Geometry check sheet. Reference: drawing and pictorial views, mm from the part's lowest x, y, z. A direction names the side the tool comes from. Coordinates: 2 decimals unless noted, no trailing zeros. Loops run counter-clockwise (first coordinate to the right, second up) from the corner with the lowest first, then second, coordinate; pieces in that order, holes last. Notation, with made-up numbers: (57, -30) -> (64, -30) arc R16 ccw to (64, 1) -> close; hole circle Ø3 at (-27.75, 43.25). An arc over 180 degrees is marked (long way). Answer as a JSON object with one key per item and string values. Group by question number.
Q1. Set-up check for the marked faces 1, 2 and 3: record each of +Z, -Z, +X, -X, +Y, -Y from which the full face is reachable in a straight line by a thin tool's end or side.
Q2. Cross-section at C-C on z = 3.2. Record the boundary of the cut face in (x, y), and give its area (3 significant figures).
Q3. Gauge pin test, flat ends, axial feed: pin 1 Ø1 at (x, z) = (6, 1.5) entering from +Y; pin 2 Ø1 at (x, z) = (2, 1) entering from +Y; pin 3 Ø2 at (y, z) = (15, 2) entering from +X. Record the tip position at first contact, or that the pin passes through.
Q4. Cross-section at D-D on z = 0.4. Record the boundary of the cut face in (x, y), and give its area (3 significant figures).
Q5. Cross-section at B-B on y = 11. Record the boundary of the cut face in (x, z).
Q6. Scan lines: L1, parallel to Z at x = 6.5, y = 8; L2, parallel to Y at x = 3.5, z = 2.4; L3, parallel to X at y = 5.75, z = 2.65. Record each from-to range of solid material in increasing order.
Q7. Cross-section at A-A on x = 3.5. Record the boundary of the cut face in (y, z), and give its area (3 significant figures).
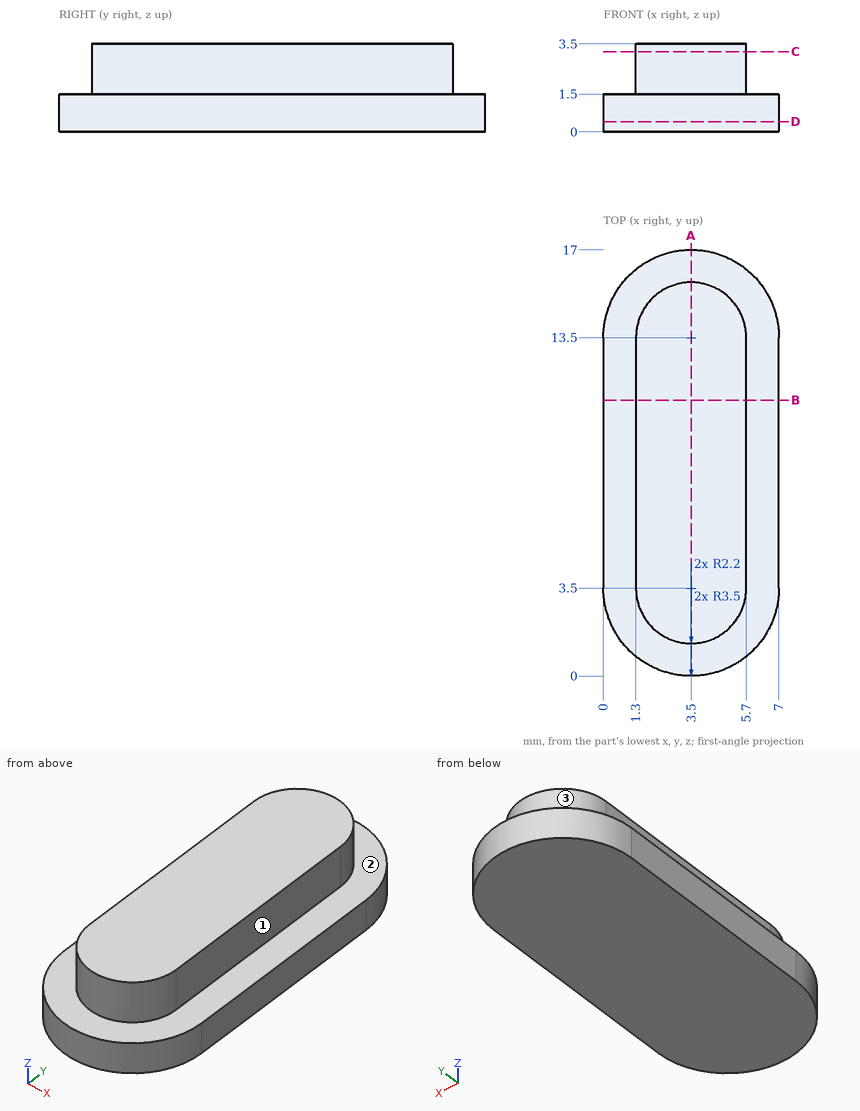
Computed values:
{
 "1": {"face 1": "+Z, +X, +Y, -Y", "face 2": "+Z", "face 3": "+Z, +Y"},
 "2": {"outline": "(1.3, 3.5) arc R2.2 ccw to (5.7, 3.5) -> (5.7, 13.5) arc R2.2 ccw to (1.3, 13.5) -> close", "area": "59.2 mm²"},
 "3": {"pin 1": "stops at y = 16.37", "pin 2": "stops at y = 16.85", "pin 3": "stops at x = 6.94"},
 "4": {"outline": "(0, 3.5) arc R3.5 ccw to (7, 3.5) -> (7, 13.5) arc R3.5 ccw to (0, 13.5) -> close", "area": "108 mm²"},
 "5": {"outline": "(0, 0) -> (7, 0) -> (7, 1.5) -> (5.7, 1.5) -> (5.7, 3.5) -> (1.3, 3.5) -> (1.3, 1.5) -> (0, 1.5) -> close"},
 "6": {"L1": "z = 0 to 1.5", "L2": "y = 1.3 to 15.7", "L3": "x = 1.3 to 5.7"},
 "7": {"outline": "(0, 0) -> (17, 0) -> (17, 1.5) -> (15.7, 1.5) -> (15.7, 3.5) -> (1.3, 3.5) -> (1.3, 1.5) -> (0, 1.5) -> close", "area": "54.3 mm²"}
}
